Source: CAD feature listing. Evaluate the final solid. Frame: model axes, mm. Give positions to 0.01 mm unless a question says otherwise; leave off trailing zeros. Order: outer loops, then holes, each group sorted by start corner. A loop starts at its lowest first (then second) coordinate and runs counter-clockwise, first axis right, second up. Notation, with made-up numbers: (55.25, 55.5) - (113.25, 55.5) arc R16 ccw to (113.25, 61.5) - close; hole circle Ø2 at (68, 17.5). An arc over 180 degrees is marked (long way). Answer as CSV lines item,"result".
```python
from build123d import *

# Parameters (mm, degrees)
SKETCH1_R            = 100
BOSS_EXTRUDE1_DEPTH  = 10
SKETCH3_W            = 60
SKETCH3_H            = 18
CUT_EXTRUDE1_DEPTH   = 142.774468788
SKETCH4_W            = 10
SKETCH4_H            = 5.88
BOSS_EXTRUDE2_DEPTH  = 2.12
SKETCH5_R            = 3.88
BOSS_EXTRUDE3_DEPTH  = 10
SKETCH6_R            = 3.88
BOSS_EXTRUDE4_DEPTH  = 10
SKETCH7_R            = 1.5
CUT_EXTRUDE2_DEPTH   = 154.436986415
BOSS_EXTRUDE5_REACH  = 219.799
SKETCH8_W            = 10
SKETCH8_H            = 5.88
BOSS_EXTRUDE6_REACH  = 219.799
SKETCH9_W            = 10
SKETCH9_H            = 5.88
BOSS_EXTRUDE8_DEPTH  = 3
CUT_EXTRUDE3_DEPTH   = 3
SKETCH22_R           = 12.5
SKETCH22_R_2         = 7.5
BOSS_EXTRUDE10_DEPTH = 5


with BuildPart() as part:
    # Sketch1 → Boss-Extrude1 (new body)
    with BuildSketch(Plane(origin=(0, 0, 0), x_dir=(1, 0, 0), z_dir=(0, 1, 0))):
        with Locations(Location((0, 0, 0), (0, 0, 270))):
            Circle(SKETCH1_R)
    extrude(amount=-BOSS_EXTRUDE1_DEPTH)

    # Sketch3 → Cut-Extrude1 (cut, through all)
    with BuildSketch(Plane(origin=(0, 0, 0), x_dir=(1, 0, 0), z_dir=(0, 1, 0))):
        with Locations((0, 100)):
            Rectangle(SKETCH3_W, SKETCH3_H)
    extrude(amount=-CUT_EXTRUDE1_DEPTH, mode=Mode.SUBTRACT)

    # Sketch4 → Boss-Extrude2 (add)
    with BuildSketch(Plane(origin=(0, 0, -91), x_dir=(-1, 0, 0), z_dir=(0, 0, -1))):
        with Locations((10, -7.06)):
            Rectangle(SKETCH4_W, SKETCH4_H)
        with Locations((-10, -7.06)):
            Rectangle(SKETCH4_W, SKETCH4_H)
    extrude(amount=BOSS_EXTRUDE2_DEPTH)


with BuildPart() as body_2:
    # Sketch5 → Boss-Extrude3 (new body)
    with BuildSketch(Plane(origin=(-5, 0, 0), x_dir=(0, 0, -1), z_dir=(1, 0, 0))):
        with Locations((97, -8)):
            Circle(SKETCH5_R)
    extrude(amount=-BOSS_EXTRUDE3_DEPTH)


with BuildPart() as body_3:
    # Sketch6 → Boss-Extrude4 (new body)
    with BuildSketch(Plane(origin=(15, 0, 0), x_dir=(0, 0, -1), z_dir=(1, 0, 0))):
        with Locations(Location((97, -8, 0), (0, 0, 90))):
            Circle(SKETCH6_R)
    extrude(amount=-BOSS_EXTRUDE4_DEPTH)


with BuildPart() as cut_extrude2_tool:
    # Sketch7 → Cut-Extrude2 (new, through all)
    with BuildSketch(Plane(origin=(15, 0, 0), x_dir=(0, 0, -1), z_dir=(1, 0, 0))):
        with Locations(Location((97, -8, 0), (0, 0, 90))):
            Circle(SKETCH7_R)
    extrude(amount=-CUT_EXTRUDE2_DEPTH)


with BuildPart() as body_2_1:
    add(body_2.part)

    # Cut-Extrude2: cut by cut_extrude2_tool
    add(cut_extrude2_tool.part, mode=Mode.SUBTRACT)

    # Sketch8 → Boss-Extrude5 (add, up to next)
    with BuildSketch(Plane(origin=(0, 0, -93.12), x_dir=(-1, 0, 0), z_dir=(0, 0, -1)), mode=Mode.PRIVATE) as boss_extrude5_sk1:
        with Locations((10, -7.06)):
            Rectangle(SKETCH8_W, SKETCH8_H)
    boss_extrude5_tool1 = extrude(boss_extrude5_sk1.sketch, amount=BOSS_EXTRUDE5_REACH, mode=Mode.PRIVATE) - body_2_1.part

    add(part.part)  # Boss-Extrude5 merges part
    add(boss_extrude5_tool1.solids().sort_by_distance((-10, -7.06, -93.12))[0])
    add(boss_extrude5_tool1.solids().sort_by_distance((-10, -7.06, -93.12))[1])


with BuildPart() as body_3_1:
    add(body_3.part)

    # Cut-Extrude2: cut by cut_extrude2_tool
    add(cut_extrude2_tool.part, mode=Mode.SUBTRACT)

    # Sketch9 → Boss-Extrude6 (add, up to next)
    with BuildSketch(Plane(origin=(0, 0, -93.12), x_dir=(-1, 0, 0), z_dir=(0, 0, -1)), mode=Mode.PRIVATE) as boss_extrude6_sk1:
        with Locations((-10, -7.06)):
            Rectangle(SKETCH9_W, SKETCH9_H)
    boss_extrude6_tool1 = extrude(boss_extrude6_sk1.sketch, amount=BOSS_EXTRUDE6_REACH, mode=Mode.PRIVATE) - body_3_1.part

    add(body_2_1.part)  # Boss-Extrude6 merges body 2
    add(boss_extrude6_tool1.solids().sort_by_distance((10, -7.06, -93.12))[0])
    add(boss_extrude6_tool1.solids().sort_by_distance((10, -7.06, -93.12))[1])

    # Sketch12 → Boss-Extrude8 (add)
    with BuildSketch(Plane(origin=(0, -10, 0), x_dir=(-1, 0, 0), z_dir=(0, -1, 0))):
        with BuildLine():
            Line((30, 95.393920142), (30, 91))
            Line((30, 91), (-30, 91))
            Line((-30, 91), (-30, 95.393920142))
            ThreePointArc((-30, 95.393920142), (0, -100), (30, 95.393920142))
        make_face()
    extrude(amount=BOSS_EXTRUDE8_DEPTH)

    # Sketch13 → Cut-Extrude3 (cut)
    with BuildSketch(Plane(origin=(0, 0, 0), x_dir=(1, 0, 0), z_dir=(0, 1, 0))):
        with BuildLine():
            Line((-30, 95.393920142), (-30, 91))
            Line((-30, 91), (30, 91))
            Line((30, 91), (30, 95.393920142))
            ThreePointArc((30, 95.393920142), (0, -100), (-30, 95.393920142))
        make_face()
    extrude(amount=-CUT_EXTRUDE3_DEPTH, mode=Mode.SUBTRACT)

    # Sketch22 → Boss-Extrude10 (add)
    with BuildSketch(Plane(origin=(0, -13, 0), x_dir=(-1, 0, 0), z_dir=(0, -1, 0))):
        with Locations((0, -100)):
            Circle(SKETCH22_R)
        with Locations((0, -100)):
            Circle(SKETCH22_R_2, mode=Mode.SUBTRACT)
    extrude(amount=-BOSS_EXTRUDE10_DEPTH)


solid = body_3_1.part
```
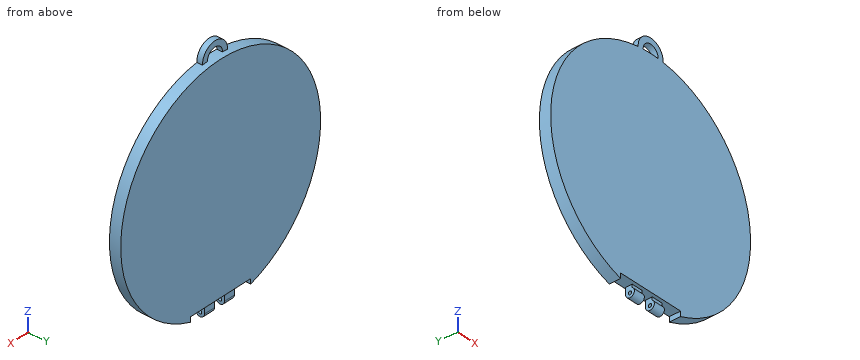
(1) Cut plane C-C (x = 23.5). Return loops of the section in (y, z), then the cut area to 3 significant figures.
Completed:
outline,"(-13, -91) - (-3, -91) - (-3, 97.2) - (-13, 97.2) - close"
area,"1,880 mm²"
(2) Ray query, line 1 (Y direction, x = 12.5, z = -97); line 2 (Z direction, x = 13.25, y = -8); line 3 (X direction, y = -7.75, z = 65). Return the intervals inside material, ascending. Write a range as from..to.
Completed:
line 1,"-11.88..-9.5, -6.5..-4.12"
line 2,"-100.88..-98.5, -95.5..99.12"
line 3,"-75.99..75.99"
(3) Contact query for flat-ended pins moving along their axis: pin 1 (5 mm diameter, centred on x = 11.5, z = -95.5, fed in from +Y); pin 2 (0.8 mm diameter, centred on x = 12.5, z = -92, fed in from -Y); pin 3 (6.5 mm diameter, centred on x = 0.5, z = 106.5, fed in from +Y). Output: stop coordinate, or through.
Completed:
pin 1,"y = -4.12"
pin 2,"y = -10"
pin 3,"y = -8"
(4) Cut plane B-B (z = 28). Return loops of the section in (x, y).
Completed:
outline,"(-96, -13) - (96, -13) - (96, -3) - (-96, -3) - close"
(5) Cut plane A-A (x = 0). Return loops of the section in (y, z).
Completed:
outline,"(-13, -91) - (-3, -91) - (-3, 100) - (-13, 100) - close; (-13, 107.5) - (-8, 107.5) - (-8, 112.5) - (-13, 112.5) - close"
